Design review of the part built by this model. Coordinates are the model's own, in mm. A direction names the side the tool comes from. Round coordinates to 2 decimals unless told otherwise and drop trailing zeros. Loops run counter-clockwise (first coordinate to the right, second up) from the corner with the lowest first, then second, coordinate; pieces in that order, holes last. Notation, with made-up numbers: (79.5, 81.25) -> (96.5, 81.25) arc R13 ccw to (96.5, 88.25) -> close; hole circle Ø6 at (-29.75, 52). An arc over 180 degrees is marked (long way). Use a Markdown table: item, result. Add a question column.
from build123d import *

# Parameters (mm, degrees)
EXTRUDE_START       = -15
EXTRUDE_1_DEPTH     = 15
EXTRUDE_START_2     = -7.5
SKETCH_2_R          = 53
SKETCH_2_R_2        = 50
EXTRUDE_2_DEPTH     = 7.5
SKETCH_3_R          = 2
CUT_EXTRUDE_1_DEPTH = 10
SKETCH_4_R          = 2
CUT_EXTRUDE_2_DEPTH = 10
SKETCH_5_R          = 2
CUT_EXTRUDE_3_DEPTH = 10
SKETCH_6_W          = 30
SKETCH_6_H          = 4.863899963
EXTRUDE_3_DEPTH     = 10
SKETCH_7_R          = 15.6
EXTRUDE_4_DEPTH     = 5
EXTRUDE_START_3     = 15
SKETCH_8_R          = 19.674554727
SKETCH_8_R_2        = 15.6
EXTRUDE_5_DEPTH     = 15
SKETCH_9_R          = 2
CUT_EXTRUDE_4_DEPTH = 131.86111959
CUT_EXTRUDE_5_DEPTH = 15


# Read off the part's stored shape, not the designer's step: 填料-伸長1
with BuildPart() as part:
    # 填料-伸長1 outline → 填料-伸長1 (new body)
    with BuildSketch(Plane(origin=(1.20571551, 0, 0), x_dir=(0, 0, -1), z_dir=(1, 0, 0)).offset(EXTRUDE_START)):
        with BuildLine():
            ThreePointArc((-28.891489898, 61.342870268), (-23.385980983, 75.484771289), (-13.891489898, 87.323632381))
            Line((-13.891489898, 87.323632381), (-20.819693129, 91.323632381))
            Line((-20.819693129, 91.323632381), (-35.819693129, 65.342870268))
            Line((-35.819693129, 65.342870268), (-28.891489898, 61.342870268))
        make_face()
        with BuildLine():
            ThreePointArc((34.915289206, 2.787811218), (19.915289206, 0.484771289), (4.915289206, 2.787811218))
            Line((4.915289206, 2.787811218), (4.915289206, -5.212188782))
            Line((4.915289206, -5.212188782), (34.915289206, -5.212188782))
            Line((34.915289206, -5.212188782), (34.915289206, 2.787811218))
        make_face()
        with BuildLine():
            ThreePointArc((53.722068311, 87.323632381), (63.216559396, 75.484771289), (68.722068311, 61.342870268))
            Line((68.722068311, 61.342870268), (75.650271541, 65.342870268))
            Line((75.650271541, 65.342870268), (60.650271541, 91.323632381))
            Line((60.650271541, 91.323632381), (53.722068311, 87.323632381))
        make_face()
    extrude(amount=EXTRUDE_1_DEPTH)

    # 草圖2 → 填料-伸長2 (add)
    with BuildSketch(Plane(origin=(1.20571551, 0, 0), x_dir=(0, 0, -1), z_dir=(1, 0, 0)).offset(EXTRUDE_START_2)):
        with Locations((19.915289206, 50.484771289)):
            Circle(SKETCH_2_R)
        with Locations((19.915289206, 50.484771289)):
            Circle(SKETCH_2_R_2, mode=Mode.SUBTRACT)
    extrude(amount=EXTRUDE_2_DEPTH)

    # 草圖3 → 除料-伸長1 (cut)
    with BuildSketch(Plane(origin=(0, 31.846099669, 55.15906265), x_dir=(1, 0, 0), z_dir=(0, 0.5000000000000088, 0.8660254037844337))):
        with Locations(Location((-6.29428449, 53.678739044, 0), (0, 0, 270))):
            Circle(SKETCH_3_R)
    extrude(amount=-CUT_EXTRUDE_1_DEPTH, mode=Mode.SUBTRACT)

    # 草圖4 → 除料-伸長2 (cut)
    with BuildSketch(Plane.XZ.offset(5.212188782)):
        with Locations(Location((-6.29428449, -19.915289206, 0), (0, 0, 270))):
            Circle(SKETCH_4_R)
    extrude(amount=-CUT_EXTRUDE_2_DEPTH, mode=Mode.SUBTRACT)

    # 草圖5 → 除料-伸長3 (cut)
    with BuildSketch(Plane(origin=(0, 49.093246046, -85.03199646), x_dir=(-1, 0, 0), z_dir=(0, 0.5000000000000044, -0.8660254037844362))):
        with Locations(Location((6.29428449, 33.763449837, 0), (0, 0, 90))):
            Circle(SKETCH_5_R)
    extrude(amount=-CUT_EXTRUDE_3_DEPTH, mode=Mode.SUBTRACT)

    # 草圖6 → 填料-伸長3 (add)
    with BuildSketch(Plane(origin=(1.20571551, 0, 0), x_dir=(0, 0, -1), z_dir=(1, 0, 0))):
        Polygon((-35.819693129, 65.342870268), (-31.6074322, 62.910920287), (-16.564749505, 88.965610996), (-20.777010434, 91.397560977), align=None)
        with Locations((19.915289206, -2.780238801)):
            Rectangle(SKETCH_6_W, SKETCH_6_H)
        Polygon((60.650271541, 91.323632381), (56.438010612, 88.8916824), (71.476544096, 62.844178335), (75.688805025, 65.276128316), align=None)
    extrude(amount=EXTRUDE_3_DEPTH)

    # 草圖7 → 填料-伸長4 (add)
    with BuildSketch(Plane(origin=(11.20571551, 0, 0), x_dir=(0, 0, -1), z_dir=(1, 0, 0))):
        Polygon((4.915289206, -0.348288819), (34.915289206, -0.348288819), (36.915289206, 40.580827444), (71.476544096, 62.844178335), (56.438010612, 88.8916824), (19.915289206, 70.114680442), (-16.6074322, 88.8916824), (-31.6074322, 62.910920287), (2.915289206, 40.669816713), align=None)
        with Locations((19.915289206, 50.484771289)):
            Circle(SKETCH_7_R, mode=Mode.SUBTRACT)
    extrude(amount=-EXTRUDE_4_DEPTH)

    # 草圖8 → 填料-伸長5 (add)
    with BuildSketch(Plane(origin=(11.20571551, 0, 0), x_dir=(0, 0, -1), z_dir=(1, 0, 0)).offset(EXTRUDE_START_3)):
        with Locations(Location((19.915289206, 50.484771289, 0), (0, 0, 209.748184736))):
            Circle(SKETCH_8_R)
        with Locations((19.915289206, 50.484771289)):
            Circle(SKETCH_8_R_2, mode=Mode.SUBTRACT)
    extrude(amount=-EXTRUDE_5_DEPTH)

    # 草圖9 → 除料-伸長4 (cut, through all)
    with BuildSketch(Plane.XY):
        with Locations((18.70571551, 50.484771289)):
            Circle(SKETCH_9_R)
    extrude(amount=-CUT_EXTRUDE_4_DEPTH, mode=Mode.SUBTRACT)

    # 草圖10 → 除料-伸長5 (cut)
    with BuildSketch(Plane(origin=(11.20571551, 0, 0), x_dir=(0, 0, -1), z_dir=(1, 0, 0))):
        Polygon((17.489472579, 14.095645642), (8.635822473, 26.014186948), (9.726460643, 3.646231166), align=None)
        Polygon((4.362874888, 72.488368192), (-15.553662135, 82.727825721), (-10.385709712, 70.780152937), align=None)
        with BuildLine():
            Line((19.981027019, 17.44940643), (26.954063356, 26.835473003))
            ThreePointArc((26.954063356, 26.835473003), (20.003346412, 25.81037369), (13.045489926, 26.785836528))
            Line((13.045489926, 26.785836528), (19.981027019, 17.44940643))
        make_face()
        Polygon((-19.953437634, 82.824030911), (-28.090922206, 68.729494185), (-14.535949667, 70.299462525), align=None)
        Polygon((22.472437105, 14.095538404), (31.188411686, 25.827689753), (30.112548712, 3.810629391), align=None)
        Polygon((-25.60433313, 64.990756457), (-7.074931027, 53.05050161), (-12.877284846, 66.464832691), align=None)
        with BuildLine():
            Line((-8.727044891, 66.945523102), (-4.084990966, 56.213663207))
            ThreePointArc((-4.084990966, 56.213663207), (-1.49739454, 62.745710311), (2.826309301, 68.283659365))
            Line((2.826309301, 68.283659365), (-8.727044891, 66.945523102))
        make_face()
        Polygon((11.843032254, -0.212188782), (28.1180014, -0.212188782), (19.980882665, 10.741777615), align=None)
        Polygon((46.747170258, 52.951758728), (65.573069111, 65.080256981), (52.642104752, 66.578515289), align=None)
        Polygon((67.856272998, 68.842471738), (59.718788426, 82.937008464), (54.300934622, 70.413073728), align=None)
        Polygon((55.237652037, 82.652928019), (35.632386961, 72.576122504), (50.15071536, 70.893942773), align=None)
        with BuildLine():
            Line((48.491885491, 67.059384335), (36.876795229, 68.405177657))
            ThreePointArc((36.876795229, 68.405177657), (41.239915747, 62.898229866), (43.874068392, 56.384817974))
            Line((43.874068392, 56.384817974), (48.491885491, 67.059384335))
        make_face()
    extrude(amount=-CUT_EXTRUDE_5_DEPTH, mode=Mode.SUBTRACT)


solid = part.part
1. For faces 1 (the face through (-6.294, 101, -20)), 2 (the face through (-1, -2, -34.915)), 3 (the face through (8.741, 14.973, -30.658)), 4 (the face through (-1.259, 75.791, -63.844)), list the 3-axis set-ups (+Z, -Z, +X, -X, +Y, -Y) from which the entire face can be reached by the end or side of a thin tool; tool diameter is ignored.
2. Consider section D-D on y = 39. State the section outline as (x, z) points.
3. Consider section A-A on x = 4. State the section outline as (y, z) points, plus the area to 3 significant figures.
4. Insertion check: P1, Ø5.5, axis at x = -1.5, z = -16.5, coming from the +Y side; P2, Ø15, axis at y = 60, z = -56, coming from the +X side; P3, Ø12, axis at x = 19, z = -32.5, coming from the -Y side; P4, Ø2, axis at x = -9, z = 2, coming from the +Y side. Each pin has a flat end and moves straight along its axis. Give the tip position at first contact, or say it passes through.
5. Consider section C-C on x = -2. State the section outline as (y, z) points, plus the area to 3 significant figures.
6. Mouldability with a two-part tool opening along Z and no side actions: class faces 5 (the face through (8.741, 67.723, -42.766)), 6 (the face through (18.81, 59.49, -37.41)), 7 (the face through (4, -0.348, -20)) as +Z half, -Z half, draft (parallel to the pull), parting line (faces both ways), or undercut.
7. Consider section B-B on z = -41. State the section outline as (x, y) points (1 decimal).
8. To check wall thickness, follow probe 1 along X at (y, z) = (86, -56); probe 2 along Z at (x, y) = (7.5, 82.5); probe 3 along Y at (x, z) = (21, -33). State the ranges of each line that lie inside material, in increasing order. Write a range as from..to.
Verdict:
| question | item | result |
|---|---|---|
| 1 | face 1 | -X, +Y |
| 1 | face 2 | -Z, -X, -Y |
| 1 | face 3 | +X, -X |
| 1 | face 4 | +X |
| 2 | outline | (-6.29, -71.66) -> (1.21, -71.66) -> (1.21, -68.58) -> (-6.29, -68.58) -> close; (-6.29, 28.75) -> (1.21, 28.75) -> (1.21, 31.83) -> (-6.29, 31.83) -> close; (6.21, -36.84) -> (11.21, -36.84) -> (11.21, -35.89) -> (26.21, -35.89) -> (26.21, -30.47) -> (6.21, -30.47) -> close; (6.21, -9.36) -> (26.21, -9.36) -> (26.21, -3.94) -> (11.21, -3.94) -> (11.21, -3) -> (6.21, -3) -> close |
| 3 | outline | (-5.21, -34.92) -> (-0.35, -34.92) -> (-0.35, -4.92) -> (-5.21, -4.92) -> close; (62.84, -71.48) -> (65.28, -75.69) -> (91.32, -60.65) -> (88.89, -56.44) -> close; (62.91, 31.61) -> (88.97, 16.56) -> (91.4, 20.78) -> (65.34, 35.82) -> close |
| 3 | area | 439 mm² |
| 4 | P1 | stops at y = 103.48 |
| 4 | P2 | stops at x = 11.21 |
| 4 | P3 | stops at y = 31.94 |
| 4 | P4 | passes through |
| 5 | outline | (-5.21, -34.92) -> (-0.35, -34.92) arc R53 ccw to (62.91, -71.44) -> (65.34, -75.65) -> (91.32, -60.65) -> (88.89, -56.44) arc R53 ccw to (88.89, 16.61) -> (91.32, 20.82) -> (65.34, 35.82) -> (62.91, 31.61) arc R53 ccw to (-0.35, -4.92) -> (-5.21, -4.92) -> close; hole (-0.21, -28.12) -> (1.02, -27.2) arc R50 ccw to (69.02, -66.35) -> (68.84, -67.86) -> (82.94, -59.72) -> (81.53, -59.11) arc R50 ccw to (81.44, 19.35) -> (82.82, 19.95) -> (68.73, 28.09) -> (68.91, 26.57) arc R50 ccw to (1, -12.74) -> (-0.21, -11.84) -> close |
| 5 | area | 1,240 mm² |
| 6 | face 5 | undercut |
| 6 | face 6 | parting line |
| 6 | face 7 | draft |
| 7 | outline | (-6.3, 1.9) -> (1.2, 1.9) -> (1.2, 5.1) -> (-6.3, 5.1) -> close; (-6.3, 95.8) -> (1.2, 95.8) -> (1.2, 99.1) -> (-6.3, 99.1) -> close; (6.2, 43.2) -> (11.2, 43.2) -> (11.2, 63.3) -> (6.2, 63.3) -> close; (6.2, 67.9) -> (11.2, 67.9) -> (11.2, 72) -> (6.2, 72) -> close; (6.2, 75.3) -> (11.2, 75.3) -> (11.2, 81) -> (6.2, 81) -> close |
| 8 | probe 1 | x = -13.79..1.21, 6.21..11.21 |
| 8 | probe 2 | z = -65.74..-59.97, -59.53..-55.17, -54.94..-44.01, 4.18..15.11, 15.46..19.81, 20.14..25.91 |
| 8 | probe 3 | y = 35.79..41.99, 58.98..65.18 |
